```python
from build123d import *

# Parameters (mm, degrees)
SKIZZE1_R                       = 1.5
AUFSATZ_LINEAR_AUSTRAGEN1_DEPTH = 3
VERRUNDUNG1_R                   = 0.1


with BuildPart() as part:
    # Skizze1 → Aufsatz-Linear austragen1 (new body)
    with BuildSketch(Plane.XY):
        Polygon((-2.309401077, 4), (-4.618802154, 0), (-2.309401077, -4), (2.309401077, -4), (4.618802154, 0), (2.309401077, 4), align=None)
        Circle(SKIZZE1_R, mode=Mode.SUBTRACT)
    extrude(amount=AUFSATZ_LINEAR_AUSTRAGEN1_DEPTH)

    # Verrundung1
    verrundung1_edges = [part.edges().sort_by_distance(p)[0] for p in [
        (-3.464101615, -2, 3),
        (0, -4, 3),
        (3.464101615, -2, 3),
        (-1.5, 0, 0),
        (-1.5, 0, 3),
        (3.464101615, 2, 3),
        (0, 4, 3),
        (3.464101615, 2, 0),
        (3.464101615, -2, 0),
        (0, -4, 0),
        (-3.464101615, 2, 3),
        (-3.464101615, -2, 0),
        (-3.464101615, 2, 0),
        (0, 4, 0),
    ]]
    fillet(verrundung1_edges, radius=VERRUNDUNG1_R)


solid = part.part
```
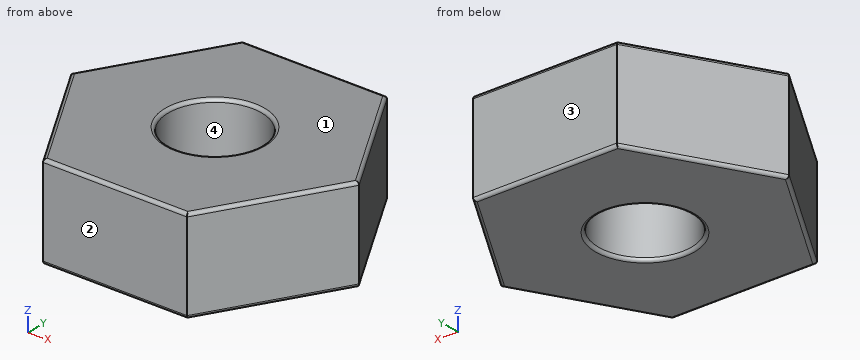
Build history of the part. All positions in model axes, mm. Face numbers are marked on the shaded views. Round coordinates to 2 decimals unless told otherwise and drop trailing zeros. Loops run counter-clockwise (first coordinate to the right, second up) from the corner with the lowest first, then second, coordinate; pieces in that order, holes last.
Item 1: Saw through at B-B (z = 0.8). List the corners of the cut face in (x, y), then the cut area to 3 significant figures.
Item 2: Two-plate mould, pull along Y, no slides. Class the marked faces 1, 2, 3 and 4: released by +Y, released by -Y, zero draft, split by the parting line, or undercut.
Item 3: Drill centre lines: line 1 along Y through (x, z) = (0, 1.6); line 2 along Z through (x, y) = (-2.5, 3.5); line 3 along Y through (x, z) = (1.25, 2.6). Where is each one in solid material? Low to high.
Item 4: Saw through at A-A (x = 0). List the corners of the cut face in (y, z), then the cut area to 3 significant figures.
Item 5: Pin check, flat tip, straight feed: P1, Ø1, axis at y = 2, z = 2.5, coming from the +X side. Stop position of the tip, or through.
Worked answers:
1. outline: (-4.62, 0) - (-2.31, -4) - (2.31, -4) - (4.62, 0) - (2.31, 4) - (-2.31, 4) - close; hole circle Ø3 at (0, 0)
1. area: 48.4 mm2
2. face 1: zero draft
2. face 2: released by -Y
2. face 3: released by +Y
2. face 4: undercut
3. line 1: y = -4 to -1.5, 1.5 to 4
3. line 2: z = 0 to 3
3. line 3: y = -4 to -0.83, 0.83 to 4
4. outline: (-4, 0.1) arc R0.1 ccw to (-3.9, 0) - (-1.6, 0) arc R0.1 ccw to (-1.5, 0.1) - (-1.5, 2.9) arc R0.1 ccw to (-1.6, 3) - (-3.9, 3) arc R0.1 ccw to (-4, 2.9) - close; (1.5, 0.1) arc R0.1 ccw to (1.6, 0) - (3.9, 0) arc R0.1 ccw to (4, 0.1) - (4, 2.9) arc R0.1 ccw to (3.9, 3) - (1.6, 3) arc R0.1 ccw to (1.5, 2.9) - close
4. area: 15.0 mm2
5. P1: stops at x = 3.75
